```python
from build123d import *

# Parameters (mm, degrees)
IZIM1_R                     = 62.2
Y_KSEKLIK_EKSTR_ZYON1_DEPTH = 10
RADYUS1_R                   = 1
IZIM2_R                     = 10
KES_EKSTR_ZYON1_DEPTH       = 10
IZIM8_R                     = 2.6
KES_EKSTR_ZYON5_DEPTH       = 10
IZIM10_R                    = 29
KES_EKSTR_ZYON7_DEPTH       = 4
M8_BO_LUKLU_DELIK1_D        = 8.4
DAIRESEL_KAPLAMA1_COUNT     = 8


with BuildPart() as part:
    # Çizim1 → Yükseklik-Ekstrüzyon1 (new body)
    with BuildSketch(Plane.XY):
        Circle(IZIM1_R)
    extrude(amount=Y_KSEKLIK_EKSTR_ZYON1_DEPTH)

    # Radyus1
    radyus1_edges = [part.edges().sort_by_distance(p)[0] for p in [
        (-62.2, 0, 0),
        (-62.2, 0, 10),
    ]]
    fillet(radyus1_edges, radius=RADYUS1_R)

    # Çizim2 → Kes-Ekstrüzyon1 (cut)
    with BuildSketch(Plane(origin=(0, 0, 0), x_dir=(-1, 0, 0), z_dir=(0, 0, -1))):
        Circle(IZIM2_R)
    extrude(amount=-KES_EKSTR_ZYON1_DEPTH, mode=Mode.SUBTRACT)

    # Çizim8 → Kes-Ekstrüzyon5 (cut)
    with BuildSketch(Plane(origin=(0, 0, 0), x_dir=(-1, 0, 0), z_dir=(0, 0, -1))):
        with Locations((16.183768006, 17.039238631)):
            Circle(IZIM8_R)
        with Locations((6.664529512, -22.535173538)):
            Circle(IZIM8_R)
        with Locations((-22.848297519, 5.495934907)):
            Circle(IZIM8_R)
    extrude(amount=-KES_EKSTR_ZYON5_DEPTH, mode=Mode.SUBTRACT)

    # Çizim10 → Kes-Ekstrüzyon7 (cut)
    with BuildSketch(Plane(origin=(0, 0, 0), x_dir=(-1, 0, 0), z_dir=(0, 0, -1))):
        Circle(IZIM10_R)
    extrude(amount=-KES_EKSTR_ZYON7_DEPTH, mode=Mode.SUBTRACT)

    # M8 Boşluklu Delik1 (through all)
    with Locations(Plane(origin=(-38.890719181, -9.35478282, 10), x_dir=(1, 0, 0), z_dir=(0, 0, 1))):
        with Locations((0, 0)):
            Hole(M8_BO_LUKLU_DELIK1_D / 2)

    # Çizim18 → M5 Boşluklu Delik1 (revolve, cut)
    with BuildSketch(Plane(origin=(0, 62.2, 5), x_dir=(0, 0, 1), z_dir=(1, 0, 0))):
        Polygon((0, 0), (0, 14.19228064), (2.65, 12.6), (2.65, 0), align=None)
    m5_bo_luklu_delik1 = revolve(axis=Axis((0, 68.55, 5), (0, -1, 0)), mode=Mode.SUBTRACT)

    # Dairesel Kaplama1: M5 Boşluklu Delik1 ×8 about axis
    dairesel_kaplama1_axis = Axis((0, 0, 10), (0, 0, -1))
    for i in range(1, DAIRESEL_KAPLAMA1_COUNT):
        add(m5_bo_luklu_delik1.rotate(dairesel_kaplama1_axis, i * 360 / DAIRESEL_KAPLAMA1_COUNT), mode=Mode.SUBTRACT)


solid = part.part
```
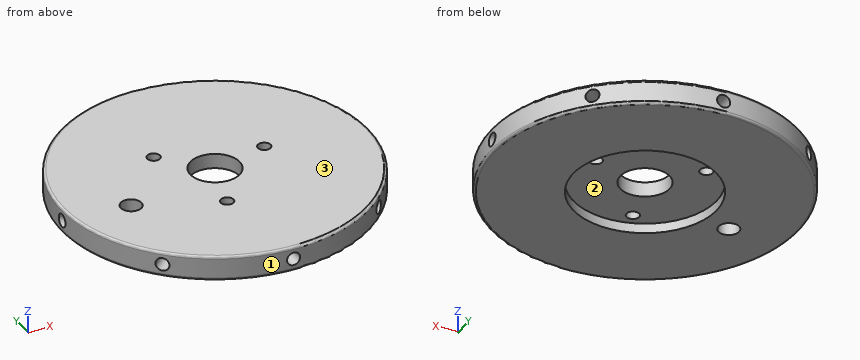
Input: part model. Units: mm. Frame: model coordinates. Face numbers are marked on the shaded views. Coordinates: 2 decimals unless noted, no trailing zeros.
1) Mould query, pull axis Y, two halves, no side actions, for the marked faces 1, 2 and 3. Classes: pulls with the +Y half, pulls with the -Y half, needs draft (parallel to the pull), parting line crosses it, or undercut.
2) Pin query (flat end, axial travel): pin 1 Ø5 at (y, z) = (28.5, 7.5) entering from +X; pin 2 Ø4 at (x, z) = (33, 1.5) entering from +Y; pin 3 Ø3 at (y, z) = (0, 5) entering from +X. Return the tip coordinate at first contact, or that it passes through.
3) Material intervals for line 1 along Y through (x, z) = (-5.5, 6.5); line 2 along X through (y, z) = (36.5, 6.5); line 3 along X through (y, z) = (13, 3.5), sorted ascending.
4) Section A-A on x = 41. State how many separate pieces and enclosed holes the cut face has, and give its area (3 significant figures).
Check result:
1. face 1: parting line crosses it
1. face 2: undercut
1. face 3: needs draft
2. pin 1: stops at x = 56.51
2. pin 2: stops at y = 53.92
2. pin 3: stops at x = 48.91
3. line 1: y = -61.96 to -24.86, -20.21 to -8.35, 8.35 to 61.96
3. line 2: x = -50.36 to -39.59, -33.57 to 33.57, 39.59 to 50.36
3. line 3: x = -60.83 to -25.92, 25.92 to 60.83
4. separate pieces: 1
4. enclosed holes: 2
4. area: 872 mm2
